The model under review builds one solid part; all positions refer to its coordinate system, in mm. Face numbers are marked on the shaded views. A direction names the side the tool comes from. Coordinates: 2 decimals unless noted, no trailing zeros. Loops run counter-clockwise (first coordinate to the right, second up) from the corner with the lowest first, then second, coordinate; pieces in that order, holes last. Notation, with made-up numbers: (45, 40) - (69, 40) arc R17 ccw to (69, 49) - close; hole circle Ø4 at (89.5, -21). An arc over 180 degrees is marked (long way). Answer in a Markdown table with one row per item. Add a question column.
(1) We need section A-A on y = -0.55. Write out the cut boundary in (x, z) (3 decimals), plus the area to 3 significant figures.
(2) For line 1 along Z through (x, y) = (-11, -0.65) (3 decimals); line 2 along X through (y, z) = (-1.25, -8), list the stretches that pass through material, from the lowest coordinate up.
(3) We need section B-B on z = -8.5. Write out the cut boundary in (x, y), plus the area to 3 significant figures.
(4) For P1, Ø0.9, axis at x = 11, y = -0.5, coming from the +Z side (3 decimals); P2, Ø1.5, axis at y = 0, z = -8, coming from the -X side; P3, Ø0.9, axis at x = -12, y = 0, coming from the -Z side (3 decimals), all flat-tipped, find the tip position at first contact; note any pin that passes through.
(5) Machinability: for the marked faces 1, 2 and 3, which of the approach directions +Z, -Z, +X, -X, +Y, -Y give a long, thin tool a straight path to every point of the face, cutting with its end or side? Answer none if there is none.
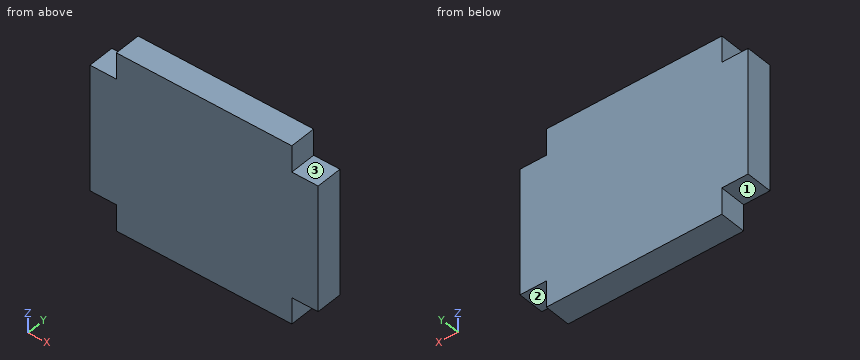
from build123d import *

# Parameters (mm, degrees)
BOSS_EXTRUDE1_DEPTH = 1.5


with BuildPart() as part:
    # Sketch1 → Boss-Extrude1 (new body, symmetric)
    with BuildSketch(Plane(origin=(0, 0, 0), x_dir=(1, 0, 0), z_dir=(0, 1, 0))):
        Polygon((-10, 10.175), (10, 10.175), (10, 7.175), (13, 7.175), (13, -7.175), (10, -7.175), (10, -10.175), (-10, -10.175), (-10, -7.175), (-13, -7.175), (-13, 7.175), (-10, 7.175), align=None)
    extrude(amount=BOSS_EXTRUDE1_DEPTH, both=True)


solid = part.part
Outcome:
| question | item | result |
|---|---|---|
| 1 | outline | (-13, -7.175) - (-10, -7.175) - (-10, -10.175) - (10, -10.175) - (10, -7.175) - (13, -7.175) - (13, 7.175) - (10, 7.175) - (10, 10.175) - (-10, 10.175) - (-10, 7.175) - (-13, 7.175) - close |
| 1 | area | 493 mm² |
| 2 | line 1 | -7.175 to 7.175 |
| 2 | line 2 | -10 to 10 |
| 3 | outline | (-10, -1.5) - (10, -1.5) - (10, 1.5) - (-10, 1.5) - close |
| 3 | area | 60.0 mm² |
| 4 | P1 | z = 7.175 |
| 4 | P2 | x = -10 |
| 4 | P3 | z = -7.175 |
| 5 | face 1 | -Z, -X, +Y, -Y |
| 5 | face 2 | -Z, +X, +Y, -Y |
| 5 | face 3 | +Z, +X, +Y, -Y |
